Can you work these out from the model? Positions are in its coordinate system, mm. A direction names the side the tool comes from. Round coordinates to 2 decimals unless told otherwise and drop trailing zeros. Order: outer loops, then holes, each group sorted by start corner. A loop starts at its lowest first (then second) coordinate and runs counter-clockwise, first axis right, second up. Notation, with made-up numbers: (-34.5, 82.5) -> (19.5, 82.5) arc R26 cw to (19.5, 97.5) -> close; hole circle Ø6 at (57.5, 62.5). An arc over 180 degrees is marked (long way). Use a Markdown table: item, result. Add a question column.
Q1. If we section it at A-A on y = 0: List the corners of the cut face in (x, z) for me.
Q2. If we section it at D-D on z = 7.5: List the corners of the cut face in (x, y) for me, plus the area to 3 significant figures.
Q3. For faces 1 (the face through (-13.887, -10.648, 1.43)), 2 (the face through (7, -7, 4)), which set-ups out of +Z, -Z, +X, -X, +Y, -Y let a thin tool reach every point of the face, with its end or its side?
Q4. I'm going to push flat-ended pins straight in: pin 1 Ø10 at (x, z) = (6.5, 7.5) entering from -Y; pin 2 Ø10 at (x, z) = (-6.5, 11.5) entering from +Y; pin 3 Ø6 at (x, z) = (-1, 6) entering from +Y; pin 4 Ø1.5 at (x, y) = (-11, 5.5) entering from -Z. Where does each tip first touch, or does it pass through?
Q5. If we section it at C-C on z = 2: List the corners of the cut face in (x, y) for me, plus the area to 3 significant figures.
Q6. I need wall thicknesses on line 1 along Z through (x, y) = (15, -3.5); line 2 along Y through (x, z) = (0, 14.75); line 3 along X through (y, z) = (3.5, 10.75). Which ranges of each line are inside material? Lowest first, please. Write a range as [from, to].
```python
from build123d import *

# Parameters (mm, degrees)
F0_R     = 17.5
F1_DEPTH = 4
F2_R     = 7
F3_DEPTH = 14
F4_SIZE  = 1.1
F5_SIZE  = 2


with BuildPart() as f1:
    # F0 (on Top) → F1 (new body)
    with BuildSketch(Plane.XY):
        Circle(F0_R)
    extrude(amount=F1_DEPTH)

    # F2 (on face) → F3 (join)
    with BuildSketch(Plane.XY.offset(4)):
        Circle(F2_R)
    extrude(amount=F3_DEPTH)

    # F4
    f4_edges = [f1.edges().sort_by_distance(p)[0] for p in [
        (-17.5, 0, 4),
    ]]
    chamfer(f4_edges, length=F4_SIZE)

    # F5
    f5_edges = [f1.edges().sort_by_distance(p)[0] for p in [
        (-7, 0, 18),
        (-7, 0, 4),
    ]]
    chamfer(f5_edges, length=F5_SIZE)


solid = f1.part
```
Answer below:
| question | item | result |
|---|---|---|
| 1 | outline | (-17.5, 0) -> (17.5, 0) -> (17.5, 2.9) -> (16.4, 4) -> (9, 4) -> (7, 6) -> (7, 16) -> (5, 18) -> (-5, 18) -> (-7, 16) -> (-7, 6) -> (-9, 4) -> (-16.4, 4) -> (-17.5, 2.9) -> close |
| 2 | outline | circle Ø14 at (0, 0) |
| 2 | area | 154 mm² |
| 3 | face 1 | +Z, -Z |
| 3 | face 2 | +Z |
| 4 | pin 1 | y = -16.9 |
| 4 | pin 2 | y = 6.84 |
| 4 | pin 3 | y = 17.38 |
| 4 | pin 4 | z = 0 |
| 5 | outline | circle Ø35 at (0, 0) |
| 5 | area | 962 mm² |
| 6 | line 1 | [0, 4] |
| 6 | line 2 | [-7, 7] |
| 6 | line 3 | [-6.06, 6.06] |
